Design review of the part built by this model. Coordinates are the model's own, in mm. Face numbers are marked on the shaded views. A direction names the side the tool comes from. Round coordinates to 2 decimals unless told otherwise and drop trailing zeros. Write each loop counter-clockwise with the first axis right and the second up, starting at its lowest first coordinate (ties: lowest second). Pieces come first, ordered by that corner, then holes. Notation, with made-up numbers: M 50,29 L 101,29 A17 ccw 101,55 Z; hole C 23.25,67.25 d2. An arc over 180 degrees is marked long. One line per question, with ' | ' between items. Start each with the question number.
Item 1: Add section D-D, the plane x = 18.5. State the section outline as (y, z) points, and give its area (3 significant figures).
Item 2: Machinability: for the marked faces 1, 2 and 3, which of the approach directions +Z, -Z, +X, -X, +Y, -Y give a long, thin tool a straight path to every point of the face, cutting with its end or side? Answer none if there is none.
Item 3: Draft analysis for pull direction Y (two halves, no side actions). For the marked faces 4 and 5, state which applies: released by +Y, released by -Y, zero draft, split by the parting line, or undercut.
Item 4: Add section B-B, the plane z = 8.5. State the section outline as (x, y) points, and give its area (3 significant figures).
Item 5: For L1, parallel to Y at x = 0, z = 77.5; L2, parallel to Z at x = -46.75, y = -70; L3, parallel to Y at x = -46, z = 80, list the stretches that pass through material, from the lowest coordinate up.
Item 6: Add section A-A, the plane x = 0. State the section outline as (y, z) points.
Item 7: Insertion check: pin 1 Ø2 at (x, y) = (56.5, 40) entering from -Z; pin 2 Ø12 at (x, y) = (42, -17) entering from +Z; pin 3 Ø5.5 at (x, z) = (-48.5, 77.5) entering from +Y; pin 4 Ø10 at (y, z) = (56, 23) entering from +X. Each pin has a flat end and moves straight along its axis. Give the tip position at first contact, or say it passes through.
Item 8: Add section C-C, the plane y = 21. State the section outline as (x, z) points.
```python
from build123d import *

# Parameters (mm, degrees)
F0_R      = 45.3
F1_DEPTH  = 75
F2_DEPTH  = 5
F3_R      = 2.5
F4_DEPTH  = 3
F5_W      = 100
F5_H      = 100
F5_R      = 48.3
F5_R_2    = 45.3
F5_R_3    = 36
F6_DEPTH  = 4
F8_DEPTH  = 3
F9_W      = 5
F9_H      = 26.435303688
F9_H_2    = 20
F10_DEPTH = 10
F12_DEPTH = 5
F14_DEPTH = 5
F15_R     = 5
F16_R     = 4.99999
F17_R     = 1.5
F18_DEPTH = 5
F20_R     = 1.5
F21_DEPTH = 5


# Not quite as in the source:
# - a fillet or chamfer is up to 0.001 mm smaller than in the source, because OpenCascade refuses the exact size


with BuildPart() as f1:
    # F0 (on Top) → F1 (new body)
    with BuildSketch(Plane.XY):
        with BuildLine():
            ThreePointArc((-7.5, 47.714148845), (-31.3898072629, -36.7092631362), (48.3, 0))
            ThreePointArc((48.3, 0), (36.7092631362, 31.3898072629), (7.5, 47.714148845))
            Line((7.5, 47.714148845), (7.5, 46.6673743725))
            Line((7.5, 46.6673743725), (-7.5, 46.6673743725))
            Line((-7.5, 46.6673743725), (-7.5, 47.714148845))
        make_face()
        Circle(F0_R, mode=Mode.SUBTRACT)
        with BuildLine():
            Line((7.5, 46.6673743725), (7.5, 47.714148845))
            ThreePointArc((7.5, 47.714148845), (0, 48.3), (-7.5, 47.714148845))
            Line((-7.5, 47.714148845), (-7.5, 46.6673743725))
            Line((-7.5, 46.6673743725), (7.5, 46.6673743725))
        make_face()
    extrude(amount=F1_DEPTH)

    # F0 (on Top) → F2 (join)
    with BuildSketch(Plane.XY):
        with BuildLine():
            ThreePointArc((-7.5, 47.714148845), (-31.3898072629, -36.7092631362), (48.3, 0))
            ThreePointArc((48.3, 0), (36.7092631362, 31.3898072629), (7.5, 47.714148845))
            Line((7.5, 47.714148845), (7.5, 46.6673743725))
            Line((7.5, 46.6673743725), (-7.5, 46.6673743725))
            Line((-7.5, 46.6673743725), (-7.5, 47.714148845))
        make_face()
        Circle(F0_R, mode=Mode.SUBTRACT)
        with BuildLine():
            Line((7.5, 46.6673743725), (7.5, 47.714148845))
            ThreePointArc((7.5, 47.714148845), (0, 48.3), (-7.5, 47.714148845))
            Line((-7.5, 47.714148845), (-7.5, 46.6673743725))
            Line((-7.5, 46.6673743725), (7.5, 46.6673743725))
        make_face()
        with BuildLine():
            ThreePointArc((-7.5, 47.714148845), (0, 48.3), (7.5, 47.714148845))
            Line((7.5, 47.714148845), (7.5, 70))
            ThreePointArc((7.5, 70), (0, 77.5), (-7.5, 70))
            Line((-7.5, 70), (-7.5, 47.714148845))
        make_face()
    extrude(amount=F2_DEPTH)

    # F3 (on face) → F4 (cut)
    with BuildSketch(Plane.XY.offset(5)):
        with Locations((0, 70)):
            Circle(F3_R)
    extrude(amount=-F4_DEPTH, mode=Mode.SUBTRACT)

    # F5 (on face) → F6 (join)
    with BuildSketch(Plane.XY.offset(75)):
        Rectangle(F5_W, F5_H)
        Circle(F5_R, mode=Mode.SUBTRACT)
        Circle(F5_R)
        Circle(F5_R_2, mode=Mode.SUBTRACT)
        Circle(F5_R_2)
        Circle(F5_R_3, mode=Mode.SUBTRACT)
    extrude(amount=F6_DEPTH)

    # F7 (on face) → F8 (join)
    with BuildSketch(Plane(origin=(0, 0, 75), x_dir=(1, 0, 0), z_dir=(0, 0, -1))):
        with BuildLine():
            Line((-68, -50), (-45.938372612, -50))
            Line((-45.938372612, -50), (-34.8247885738, -50))
            ThreePointArc((-34.8247885738, -50), (-30.5975043414, -47.6702187211), (-30.3096791752, -42.8520272073))
            Line((-30.3096791752, -42.8520272073), (-45.938372612, -10))
            Line((-45.938372612, -10), (-68, -10))
            ThreePointArc((-68, -10), (-71.5355339059, -11.4644660941), (-73, -15))
            Line((-73, -15), (-73, -45))
            ThreePointArc((-73, -45), (-71.5355339059, -48.5355339059), (-68, -50))
        make_face()
        with BuildLine():
            Line((68, -10), (45.938372612, -10))
            Line((45.938372612, -10), (30.3096791752, -42.8520272073))
            ThreePointArc((30.3096791752, -42.8520272073), (30.5975043414, -47.6702187211), (34.8247885738, -50))
            Line((34.8247885738, -50), (45.938372612, -50))
            Line((45.938372612, -50), (68, -50))
            ThreePointArc((68, -50), (71.5355339059, -48.5355339059), (73, -45))
            Line((73, -45), (73, -15))
            ThreePointArc((73, -15), (71.5355339059, -11.4644660941), (68, -10))
        make_face()
    extrude(amount=F8_DEPTH)

    # F9 (on face) → F10 (join)
    with BuildSketch(Plane(origin=(0, 0, 75), x_dir=(1, 0, 0), z_dir=(0, 0, -1))):
        with Locations((47.5, 36.782348156)):
            Rectangle(F9_W, F9_H)
        with Locations((47.5, 60)):
            Rectangle(F9_W, F9_H_2)
    extrude(amount=F10_DEPTH)

    # F11 (on face) → F12 (cut, through all)
    with BuildSketch(Plane.YZ.offset(50)):
        with BuildLine():
            ThreePointArc((-23.564696312, 75), (-26.3246425928, 68.0971789948), (-33.0828763545, 65))
            Line((-33.0828763545, 65), (-23.564696312, 65))
            Line((-23.564696312, 65), (-23.564696312, 75))
        make_face()
    extrude(amount=-F12_DEPTH, mode=Mode.SUBTRACT)

    # F13 (on face) → F14 (join)
    with BuildSketch(Plane.YZ.offset(50)):
        Polygon((-70, 65), (-70, 75), (-65, 75), (-65, 85), (-75, 85), (-75, 65), align=None)
    extrude(amount=-F14_DEPTH)

    # F15
    f15_edges = [f1.edges().sort_by_distance(p)[0] for p in [
        (47.5, -75, 65),
    ]]
    fillet(f15_edges, radius=F15_R)

    # F16 (radius 5 in the source; OpenCascade refuses exactly that, so slightly less here)
    f16_edges = [f1.edges().sort_by_distance(p)[0] for p in [
        (47.5, -75, 85),
        (47.5, -65, 85),
    ]]
    fillet(f16_edges, radius=F16_R)

    # F17 (on face) → F18 (cut, through all)
    with BuildSketch(Plane.YZ.offset(50)):
        with Locations((-70, 80)):
            Circle(F17_R)
    extrude(amount=-F18_DEPTH, mode=Mode.SUBTRACT)

    # F20 (on offset) → F21 (join)
    with BuildSketch(Plane(origin=(-50, 0, 0), x_dir=(0, -1, 0), z_dir=(-1, 0, 0))):
        with BuildLine():
            Line((75, 70), (75, 80))
            ThreePointArc((75, 80), (70, 85), (65, 80))
            Line((65, 80), (65, 75))
            Line((65, 75), (50, 75))
            Line((50, 75), (23.564696312, 75))
            ThreePointArc((23.564696312, 75), (26.3246425928, 68.0971789948), (33.0828763545, 65))
            Line((33.0828763545, 65), (70, 65))
            ThreePointArc((70, 65), (73.5355339059, 66.4644660941), (75, 70))
        make_face()
        with Locations((70, 80)):
            Circle(F20_R, mode=Mode.SUBTRACT)
    extrude(amount=-F21_DEPTH)


solid = f1.part
```
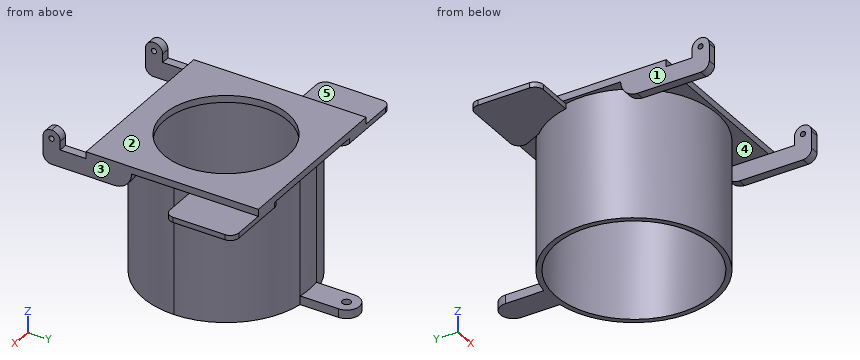
Computed values:
1) outline: M -50,75 L -44.62,75 L -44.62,0 L -41.35,0 L -41.35,75 L -30.88,75 L -30.88,79 L -50,79 Z; M 30.88,75 L 41.35,75 L 41.35,0 L 44.62,0 L 44.62,75 L 50,75 L 50,79 L 30.88,79 Z | area: 643 mm^2
2) face 1: +Z, -X, -Y | face 2: +Z, +X, -X, +Y | face 3: +Z, +X, -Y
3) face 4: undercut | face 5: zero draft
4) outline: C 0,0 d96.6; hole C 0,0 d90.6 | area: 882 mm^2
5) L1: y = -50 to -36, 36 to 50 | L2: z = 65 to 78.5, 81.5 to 85 | L3: y = -75 to -71.5, -68.5 to -65
6) outline: M -50,75 L -48.3,75 L -48.3,0 L -45.3,0 L -45.3,75 L -36,75 L -36,79 L -50,79 Z; M 36,75 L 45.3,75 L 45.3,0 L 77.5,0 L 77.5,5 L 72.5,5 L 72.5,2 L 67.5,2 L 67.5,5 L 48.3,5 L 48.3,75 L 50,75 L 50,79 L 36,79 Z
7) pin 1: stops at z = 72 | pin 2: stops at z = 79 | pin 3: stops at y = 50 | pin 4: passes through
8) outline: M -73,72 L -43.5,72 L -43.5,0 L -40.14,0 L -40.14,75 L -29.24,75 L -29.24,79 L -50,79 L -50,75 L -73,75 Z; M 29.24,75 L 40.14,75 L 40.14,0 L 43.5,0 L 43.5,72 L 73,72 L 73,75 L 50,75 L 50,79 L 29.24,79 Z
